```python
from build123d import *

# Parameters (mm, degrees)
SKETCH1_R           = 38.1
SKETCH1_W           = 127
SKETCH1_H           = 76.2
BOSS_EXTRUDE1_DEPTH = 12.7
SKETCH2_R           = 4.7625
CUT_EXTRUDE2_DEPTH  = 113.430244289


with BuildPart() as part:
    # Sketch1 → Boss-Extrude1 (new body)
    with BuildSketch(Plane(origin=(0, 0, 0), x_dir=(1, 0, 0), z_dir=(0, 1, 0))):
        with Locations((-66.912665097, 0)):
            Circle(SKETCH1_R)
        with Locations((60.087334903, 0)):
            Circle(SKETCH1_R)
        with Locations((-3.412665097, 0)):
            Rectangle(SKETCH1_W, SKETCH1_H)
    extrude(amount=BOSS_EXTRUDE1_DEPTH)

    # Sketch2 → Cut-Extrude2 (cut, through all)
    with BuildSketch(Plane(origin=(0, 12.7, 0), x_dir=(1, 0, 0), z_dir=(0, 1, 0))):
        with Locations(Location((-66.912665097, 0, 0), (0, 0, 270))):
            Circle(SKETCH2_R)
        with Locations(Location((60.087334903, 0, 0), (0, 0, 270))):
            Circle(SKETCH2_R)
    extrude(amount=-CUT_EXTRUDE2_DEPTH, mode=Mode.SUBTRACT)


solid = part.part
```
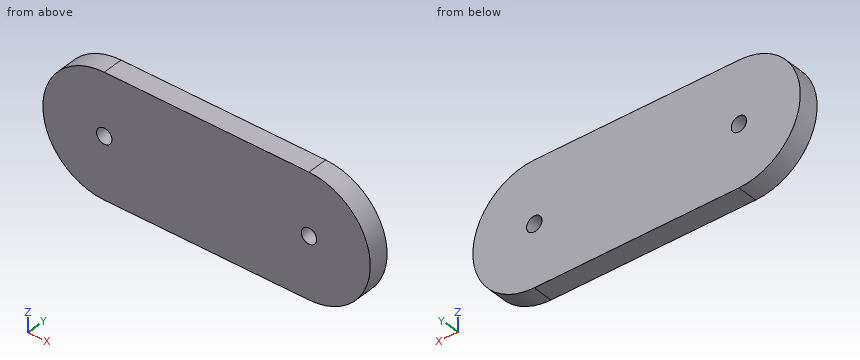
CAD build for the part. Positions are in the model's coordinates, mm. Give positions to 0.01 mm unless a question says otherwise; leave off trailing zeros. Loops run counter-clockwise (first coordinate to the right, second up) from the corner with the lowest first, then second, coordinate; pieces in that order, holes last. Notation, with made-up numbers: (59.5, 16) -> (115.5, 16) arc R20 ccw to (115.5, 45) -> close; hole circle Ø8 at (-23.5, -32). An arc over 180 degrees is marked (long way). Use a Markdown table: item, result.
1. Slice it at A-A (z = 0). List the corners of the cut face in (x, y).
Check result:
| item | result |
|---|---|
| outline | (-105.01, 0) -> (-71.68, 0) -> (-71.68, 12.7) -> (-105.01, 12.7) -> close; (-62.15, 0) -> (55.32, 0) -> (55.32, 12.7) -> (-62.15, 12.7) -> close; (64.85, 0) -> (98.19, 0) -> (98.19, 12.7) -> (64.85, 12.7) -> close |
2. Slice it at D-D (z = 20.5). List the corners of the cut face in (x, y).
Check result:
| item | result |
|---|---|
| outline | (-99.03, 0) -> (92.2, 0) -> (92.2, 12.7) -> (-99.03, 12.7) -> close |
3. Wall check: L1, parallel to X at y = 7, z = 0; L2, parallel to X at y = 4.5, z = -3; L3, parallel to X at y = 10.25, z = 33. Give the ranges that are in metal, low to high. Write a range as [from, to].
Check result:
| item | result |
|---|---|
| L1 | x = [-105.01, -71.68], [-62.15, 55.32], [64.85, 98.19] |
| L2 | x = [-104.89, -70.61], [-63.21, 56.39], [63.79, 98.07] |
| L3 | x = [-85.95, 79.13] |
4. Slice it at C-C (x = 69). List the corners of the cut face in (y, z), plus the area to 3 significant figures.
Check result:
| item | result |
|---|---|
| outline | (0, -37.04) -> (12.7, -37.04) -> (12.7, 37.04) -> (0, 37.04) -> close |
| area | 941 mm^2 |
5. Flat gauge pins, fed straight in: pin 1 (4 mm diameter, centred on y = 3.5, z = 12.5, fed in from +X); pin 2 (5 mm diameter, centred on y = 9.5, z = 25.5, fed in from +X); pin 3 (5 mm diameter, centred on y = 6.5, z = 24.5, fed in from +X). Where does each tip first touch, or does it go through?
Check result:
| item | result |
|---|---|
| pin 1 | stops at x = 96.71 |
| pin 2 | stops at x = 90.46 |
| pin 3 | stops at x = 91.19 |
6. Slice it at B-B (y = 2). List the corners of the cut face in (x, z) (1 decimal), plus the area to 3 significant figures.
Check result:
| item | result |
|---|---|
| outline | (-66.9, -38.1) -> (60.1, -38.1) arc R38.1 ccw to (60.1, 38.1) -> (-66.9, 38.1) arc R38.1 ccw to start; hole circle Ø9.5 at (-66.9, 0); hole circle Ø9.5 at (60.1, 0) |
| area | 14,100 mm^2 |
